Work out the finished part from the listing and answer in its coordinate system (mm). A direction names the side the tool comes from. Coordinates: 2 decimals unless noted, no trailing zeros. Write each loop counter-clockwise with the first axis right and the second up, starting at its lowest first coordinate (ties: lowest second). Pieces come first, ordered by that corner, then holes. Notation, with made-up numbers: (38.25, 88.5) - (83.25, 88.5) arc R20 cw to (83.25, 117.5) - close; hole circle Ø6 at (-39.5, 8.5). An arc over 180 degrees is marked (long way). One line per item, written item: value.
```python
from build123d import *

# Parameters (mm, degrees)
F0_R           = 11
F0_R_2         = 3.8
F0_R_3         = 3.3
F1_DEPTH       = 2.5
F2_DEPTH       = 1
F3_D           = 0.8
F3_CSINK_D     = 1.6
F3_CSINK_ANGLE = 135


with BuildPart() as f1:
    # F0 (on Top) → F1 (new body)
    with BuildSketch(Plane.XY):
        Circle(F0_R)
        Circle(F0_R_2, mode=Mode.SUBTRACT)
        Circle(F0_R_2)
        Circle(F0_R_3, mode=Mode.SUBTRACT)
    extrude(amount=F1_DEPTH)

    # F0 (on Top) → F2 (join)
    with BuildSketch(Plane.XY):
        Circle(F0_R_2)
        Circle(F0_R_3, mode=Mode.SUBTRACT)
    extrude(amount=-F2_DEPTH)

    # F3 (through all)
    with Locations(Plane(origin=(0, 0, 0), x_dir=(1, 0, 0), z_dir=(0, 0, -1))):
        with Locations((0, 7), (7, 0), (0, -7), (-7, 0)):
            CounterSinkHole(F3_D / 2, F3_CSINK_D / 2, counter_sink_angle=F3_CSINK_ANGLE)


solid = f1.part
```
Item 1: Given pin 1 (2 mm diameter, centred on x = 8, z = 0, fed in from +Y), flat-ended and moving along its own axis, determine where the tip first touches the part or whether it passes through.
Evaluation:
pin 1: stops at y = 8.49
Item 2: Determine the mould class of faces 3 (the face through (-3, 2, -1)), 4 (the face through (-6.705, -0.27, 1.349)), 5 (the face through (-3.796, 0.167, -0.493)) for opening direction X: +X half, -X half, draft (parallel to the pull), parting line (faces both ways), or undercut.
Evaluation:
face 3: draft
face 4: undercut
face 5: parting line
Item 3: Consider probe 1 along Y at (x, z) = (0, 1.25); probe 2 along X at (y, z) = (-0.25, 2.25); probe 3 along Z at (x, y) = (-3, -5.25). Determine where each line is inside the solid, lowest interval first.
Evaluation:
probe 1: y = -11 to -7.4, -6.6 to -3.3, 3.3 to 6.6, 7.4 to 11
probe 2: x = -11 to -7.31, -6.69 to -3.29, 3.29 to 6.69, 7.31 to 11
probe 3: z = 0 to 2.5
Item 4: Section A-A, the plane y = 0 is taken. Determine the outline of the cut face in (x, z).
Evaluation:
outline: (-11, 0) - (-7.8, 0) - (-7.4, 0.17) - (-7.4, 2.5) - (-11, 2.5) - close; (-6.6, 0.17) - (-6.2, 0) - (-3.8, 0) - (-3.8, -1) - (-3.3, -1) - (-3.3, 2.5) - (-6.6, 2.5) - close; (3.3, -1) - (3.8, -1) - (3.8, 0) - (6.2, 0) - (6.6, 0.17) - (6.6, 2.5) - (3.3, 2.5) - close; (7.4, 0.17) - (7.8, 0) - (11, 0) - (11, 2.5) - (7.4, 2.5) - close
Item 5: Which of the six approach directions +Z, -Z, +X, -X, +Y, -Y give full straight-line access (tool end or side, diameter ignored) to faces 1 (the face through (0, -5, 0)), 2 (the face through (7.295, -0.27, 1.349))?
Evaluation:
face 1: -Z
face 2: +Z, -Z
Item 6: Section C-C, the plane x = -7 is taken. Determine the outline of the cut face in (y, z).
Evaluation:
outline: (-8.49, 0) - (-0.8, 0) - (-0.4, 0.17) - (-0.4, 2.5) - (-8.49, 2.5) - close; (0.4, 0.17) - (0.8, 0) - (8.49, 0) - (8.49, 2.5) - (0.4, 2.5) - close
Item 7: Section D-D, the plane y = -2.25 is taken. Determine the outline of the cut face in (x, z).
Evaluation:
outline: (-10.77, 0) - (-3.06, 0) - (-3.06, -1) - (-2.41, -1) - (-2.41, 2.5) - (-10.77, 2.5) - close; (2.41, -1) - (3.06, -1) - (3.06, 0) - (10.77, 0) - (10.77, 2.5) - (2.41, 2.5) - close
